Source: three-view drawing plus pictorial views. Frame: mm from the lowest corner of the part. A direction names the side the tool comes from. Give positions to 0.01 mm unless a question says otherwise; leave off trailing zeros. Order: outer loops, then holes, each group sorted by start corner. A loop starts at its lowest first (then second) coordinate and runs counter-clockwise, first axis right, second up. Notation, with made-up numbers: (67.5, -30) - (99.5, -30) arc R17 ccw to (99.5, -23) - close; hole circle Ø3 at (-7.5, 12.25). An arc over 180 degrees is marked (long way). Use one line per item in the form item = value.
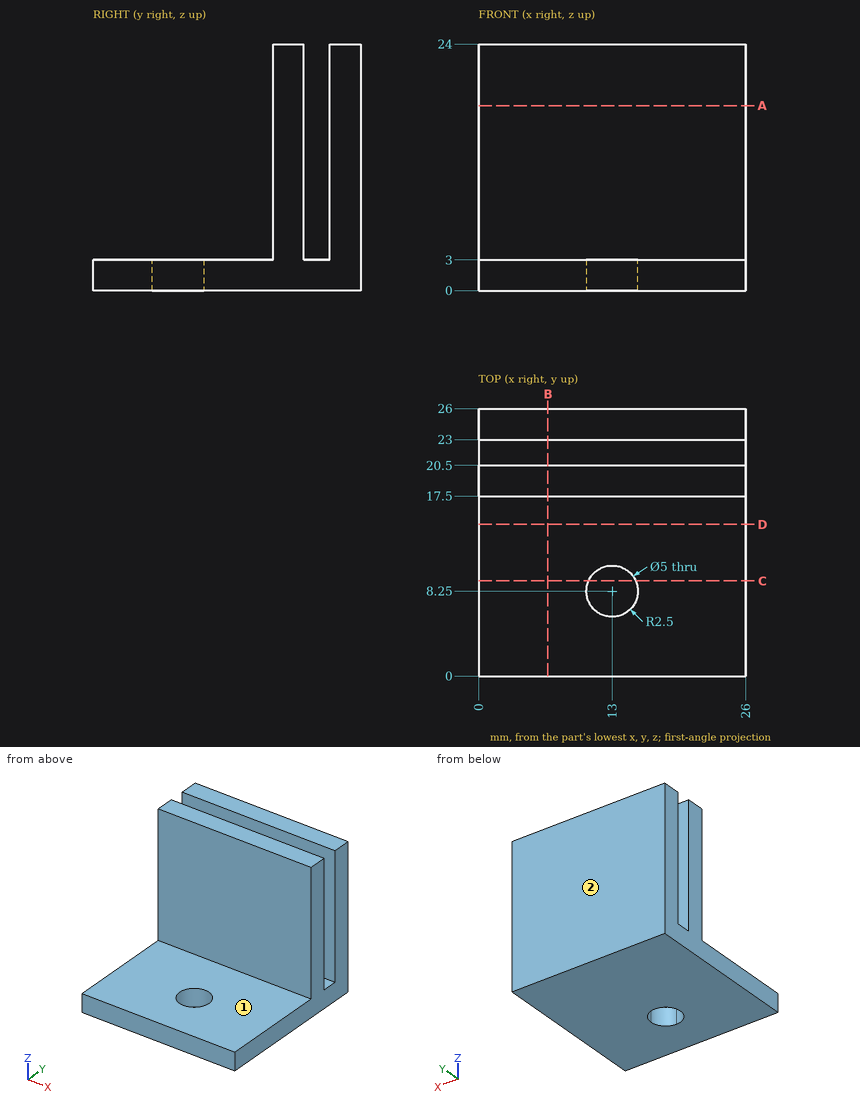
(1) Reachability of the marked faces 1 and 2 from +Z, -Z, +X, -X, +Y, -Y: full face, straight path, thin tool, end or side. Return the list, or none.
Computed values:
face_1 = +Z, +X, -X, -Y
face_2 = +Z, -Z, +X, -X, +Y
(2) Contact query for flat-ended pins moving along their axis: pin 1 Ø6.5 at (x, z) = (14.5, 17.5) entering from -Y; pin 2 Ø5 at (y, z) = (14, 20) entering from -X. Output: stop coordinate, or through.
Computed values:
pin_1 = 17.5
pin_2 = through
(3) Ray query, line 1 along Y through (x, z) = (13, 0.8); line 2 along X through (y, z) = (8.25, 1.55); line 3 along Y through (x, z) = (11.25, 21.5). Return the intervals inside material, ascending.
Computed values:
line_1 = 0 to 5.75, 10.75 to 26
line_2 = 0 to 10.5, 15.5 to 26
line_3 = 17.5 to 20.5, 23 to 26
(4) Cut plane C-C on y = 9.25. Output: boundary loops of the cut face in (x, z).
Computed values:
outline = (0, 0) - (10.71, 0) - (10.71, 3) - (0, 3) - close; (15.29, 0) - (26, 0) - (26, 3) - (15.29, 3) - close
(5) Cut plane A-A on z = 18. Output: boundary loops of the cut face in (x, y), plus the area to 3 significant figures.
Computed values:
outline = (0, 17.5) - (26, 17.5) - (26, 20.5) - (0, 20.5) - close; (0, 23) - (26, 23) - (26, 26) - (0, 26) - close
area = 156 mm²
(6) Cut plane B-B on x = 6.75. Output: boundary loops of the cut face in (y, z).
Computed values:
outline = (0, 0) - (26, 0) - (26, 24) - (23, 24) - (23, 3) - (20.5, 3) - (20.5, 24) - (17.5, 24) - (17.5, 3) - (0, 3) - close
(7) Cut plane D-D on y = 14.75. Output: boundary loops of the cut face in (x, z).
Computed values:
outline = (0, 0) - (26, 0) - (26, 3) - (0, 3) - close
